Autodesk Inventor part; units mm, degrees
ref_plane "YZ Plane" through (0, 0, 0) normal (1, 0, 0) x (0, 1, 0)
ref_plane "XZ Plane" through (0, 0, 0) normal (0, 1, 0) x (-1, 0, 0)
ref_plane "XY Plane" through (0, 0, 0) normal (0, 0, 1) x (1, 0, 0)
sketch "スケッチ2" plane through (-42.95, -23.5, 0) normal (0, -1, 0) x (1, 0, 0)
  line L0 (0, 0) -> (25.9, 5) construction
  line L1 (0, 5) -> (25.9, 5)
  line L2 (12.95, 5) -> (12.95, 0) construction
  line L3 (0, 0) -> (25.9, 0)
  line L4 (0, 0) -> (0, 5)
  line L5 (0, 2.5) -> (25.9, 2.5) construction
  line L6 (25.9, 0) -> (25.9, 5)
  point P0 (42.95, 0)
  point P1 (2.95, 2.5)
  point P2 (22.95, 2.5)
  dimension "d176" = 20
sketch "スケッチ1" plane through (0, 0, 0) normal (0, 0, 1) x (1, 0, 0)
  line L0 (-72.5, 26.5) -> (-45, 26.5) construction
  line L1 (72.5, 26.5) -> (72.5, 10.5) construction
  line L2 (-72.5, -26.5) -> (-72.5, 10.5)
  line L3 (-72.5, 26.5) -> (72.5, -26.5) construction
  line L4 (72.5, 26.5) -> (-72.5, -26.5) construction
  line L5 (2.5, 26.5) -> (2.5, 10.5)
  line L6 (2.5, 10.5) -> (4.6, 10.5) construction
  line L7 (2.5, 26.5) -> (72.5, 26.5) construction
  line L8 (72.5, 10.5) -> (72.5, -26.5)
  line L9 (70, 10.5) -> (70, -26) construction
  circle A0 centre (67.5, 5.5) radius 1.55
  line L10 (-31.25, 26.5) -> (-31.25, 31.5)
  line L11 (-31.25, 31.5) -> (-11.25, 31.5)
  line L12 (-11.25, 31.5) -> (-11.25, 26.5)
  line L13 (-31.25, 26.5) -> (-11.25, 26.5) construction
  line L14 (-11.25, 26.5) -> (-9.15, 26.5) construction
  arc A1 (-33.35, 26.5) -> (-31.25, 26.5) centre (-32.3, 26.5) ccw
  arc A2 (-11.25, 26.5) -> (-9.15, 26.5) centre (-10.2, 26.5) ccw
  line L15 (-33.35, 26.5) -> (-31.25, 26.5) construction
  line L16 (-9.15, 26.5) -> (2.5, 26.5)
  line L17 (-45.05, -23.5) -> (-42.95, -23.5) construction
  arc A3 (-42.95, -23.5) -> (-45.05, -23.5) centre (-44, -23.5) ccw
  arc A4 (-14.95, -23.5) -> (-17.05, -23.5) centre (-16, -23.5) ccw
  line L18 (-42.95, -23.5) -> (-17.05, -23.5)
  line L19 (-17.05, -23.5) -> (-14.95, -23.5) construction
  line L20 (15, -23.5) -> (45, -23.5) construction
  line L21 (45, -23.5) -> (45, -25) construction
  line L22 (45, -25) -> (15, -25) construction
  line L23 (15, -25) -> (15, -23.5) construction
  line L24 (15, -23.5) -> (45, -25) construction
  line L25 (45, -23.5) -> (15, -25) construction
  line L26 (14.95, -23.45) -> (45.05, -23.45)
  line L27 (45.05, -23.45) -> (45.05, -25.05) construction
  line L28 (45.05, -25.05) -> (14.95, -25.05)
  line L29 (14.95, -25.05) -> (14.95, -23.45) construction
  line L30 (14.95, -23.45) -> (45.05, -25.05) construction
  line L31 (45.05, -23.45) -> (14.95, -25.05) construction
  line L32 (-45, -23.5) -> (-45, -26.5) construction
  line L33 (-15, -23.5) -> (-15, -26.5) construction
  line L34 (72.5, -8) -> (-72.5, -8) construction
  line L35 (70, -0.5) -> (67.5, -0.5) construction
  line L36 (67.5, -0.5) -> (67.5, -15.5) construction
  line L37 (67.5, -15.5) -> (70, -15.5) construction
  line L38 (70, -15.5) -> (70, -0.5) construction
  line L39 (70, -0.5) -> (67.5, -15.5) construction
  line L40 (67.5, -0.5) -> (70, -15.5) construction
  line L41 (67.45, -0.45) -> (70.05, -0.45)
  line L42 (70.05, -0.45) -> (70.05, -2.55) construction
  line L43 (70.05, -15.55) -> (67.45, -15.55)
  line L44 (67.45, -15.55) -> (67.45, -13.45) construction
  line L45 (67.45, -0.45) -> (70.05, -15.55) construction
  line L46 (70.05, -0.45) -> (67.45, -15.55) construction
  arc A5 (67.45, -0.45) -> (67.45, -2.55) centre (67.45, -1.5) ccw
  arc A6 (70.05, -2.55) -> (70.05, -0.45) centre (70.05, -1.5) ccw
  arc A7 (67.45, -13.45) -> (67.45, -15.55) centre (67.45, -14.5) ccw
  arc A8 (70.05, -15.55) -> (70.05, -13.45) centre (70.05, -14.5) ccw
  line L47 (67.45, -2.55) -> (67.45, -0.45) construction
  line L48 (67.45, -13.45) -> (67.45, -2.55)
  line L49 (70.05, -13.45) -> (70.05, -15.55) construction
  line L50 (70.05, -2.55) -> (70.05, -13.45)
  arc A9 (14.95, -23.45) -> (14.95, -25.05) centre (14.95, -24.25) ccw
  arc A10 (45.05, -25.05) -> (45.05, -23.45) centre (45.05, -24.25) ccw
  circle A11 centre (67.5, -21.5) radius 1.55
  line L51 (-72.5, -26.5) -> (-62.5, -26.5) construction
  line L52 (-15, -26.5) -> (72.5, -26.5)
  line L53 (-45, -26.5) -> (-15, -26.5) construction
  line L54 (-70, 26) -> (-70, -26.5) construction
  line L55 (-65, 26.5) -> (-65, -26.5) construction
  arc A12 (2.5, 10.5) -> (4.6, 10.5) centre (3.55, 10.5) ccw
  line L56 (4.6, 10.5) -> (72.5, 10.5)
  circle A13 centre (67.5, 5.5) radius 3
  circle A14 centre (67.5, -21.5) radius 3
  line L57 (2.5, 5.5) -> (2.5, -18.5)
  line L58 (2.5, -18.5) -> (51.8308, -18.5)
  line L59 (51.8308, -18.5) -> (6.5905, 5.5)
  line L60 (17.2597, 5.5) -> (62.5, 5.5)
  line L61 (62.5, 5.5) -> (62.5, -18.5)
  line L62 (62.5, -18.5) -> (17.2597, 5.5)
  line L63 (-62.5, -18.5) -> (-6.9355, -18.5)
  line L64 (-6.9355, -18.5) -> (-42.1079, 5.5)
  line L65 (-2.5, 21.5) -> (-2.5, -15.4734)
  line L66 (-2.5, -15.4734) -> (-40, 10.1148)
  line L67 (2.5, 10.5) -> (2.5, -26.5) construction
  line L68 (6.5905, 5.5) -> (2.5, 5.5)
  line L69 (2.5, 10.5) -> (72.2455, -26.5) construction
  circle A15 centre (-67.5, -29) radius 1.25
  circle A16 centre (-67.5, -29) radius 3
  circle A17 centre (-67.5, -2) radius 1.5
  circle A18 centre (-67.5, 3) radius 1.5
  circle A19 centre (-67.5, 8) radius 1.5
  line L70 (-67.5, 26.5) -> (-67.5, -26.5) construction
  line L71 (-45.05, -23.5) -> (-45.05, -26.5)
  line L72 (-14.95, -23.5) -> (-14.95, -26.5)
  line L73 (-45, 26.5) -> (-45, 21.5)
  line L74 (-45, 10.5) -> (-72.5, 10.5)
  line L75 (-62.5, 5.5) -> (-42.1079, 5.5)
  line L76 (-40, 21.5) -> (-40, 10.1148)
  line L77 (-72.5, -26.5) -> (-72.5, -34)
  line L78 (-72.5, -34) -> (-62.5, -34)
  line L79 (-62.5, -26.5) -> (-62.5, -34)
  line L80 (-62.5, -26.5) -> (-45, -26.5)
  line L81 (-45, 26.5) -> (-33.35, 26.5)
  line L82 (-45, 21.5) -> (-45, 10.5)
  line L83 (-62.5, 5.5) -> (-62.5, -18.5)
  line L84 (-2.5, -18.5) -> (-45, 10.5) construction
  line L85 (-45.05, 21.5) -> (-45, 21.5)
  line L86 (-40, 21.5) -> (-2.5, 21.5)
  line L87 (-72.5, 10.5) -> (-72.5, 26.5) construction
  point P0 (0, 0)
  point P1 (30, -24.25)
  point P2 (68.75, -8)
  point P3 (-60, 14.6054)
  point P4 (-46.25, 11.0112)
  point P5 (-54.1904, 10.5)
  point P6 (-45.5266, 10.5)
  dimension "d0" = 145
  dimension "d1" = 53
  dimension "d2" = 75
  dimension "d3" = 16
  dimension "d4" = 2.5
  dimension "d5" = 3.1
  dimension "d6" = 2.5
  dimension "d7" = 5
  dimension "d12" = 20
  dimension "d14" = 5
  dimension "d15" = 1.05
  dimension "d16" = 1.05
  dimension "d17" = 70
  dimension "d55" = 1.05
  dimension "d56" = 1.05
  dimension "d74" = 37
  dimension "d107" = 30
  dimension "d108" = 1.5
  dimension "d109" = 0.05
  dimension "d110" = 0.05
  dimension "d116" = 30
  dimension "d124" = 15
  dimension "d125" = 0.05
  dimension "d126" = 0.05
  dimension "d127" = 1.05
  dimension "d128" = 1.05
  dimension "d129" = 1.05
  dimension "d130" = 1.05
  dimension "d132" = 30
  dimension "d134" = 3
  dimension "d135" = 2.5
  dimension "d146" = 5
  dimension "d147" = 20
  dimension "d152" = 1.05
  dimension "d169" = 6
  dimension "d186" = 5
  dimension "d187" = 5
  dimension "d190" = 8
  dimension "d192" = 5
  dimension "d193" = 5
  dimension "d196" = 2.5
  dimension "d200" = 2.5
  dimension "d201" = 6
  dimension "d205" = 2.5
  dimension "d206" = 3
  dimension "d207" = 3
  dimension "d208" = 3
  dimension "d209" = 2.5
  dimension "d211" = 5
  dimension "d212" = 5
  dimension "d213" = 0.05
  dimension "d214" = 0.05
  dimension "d215" = 2.5
  dimension "d216" = 5
  dimension "d217" = 2.5
  dimension "d220" = 18.5
  dimension "d222" = 16
  dimension "d225" = 13.75
  dimension "d226" = 27.5
  dimension "d227" = 5
  dimension "d228" = 5
  dimension "d233" = 7.5
  dimension "d234" = 2.5
  dimension "d235" = 2.5
extrude "押し出し1" add sketch "スケッチ1" along normal blind 5 contours L2 L74 L82 L73 L81 A1 L10 L11 L12 A2 L16 L5 A12 L56 L8 L52 L72 A4 L18 A3 L71 L80 L79 L78 L77
extrude "押し出し2" add sketch "スケッチ1" along normal blind 2 contours A13 | A14 | A16
hole "穴1" at (-40, -23.5, 2.5) at (-20, -23.5, 2.5) direction (0, 1, 0) diameter 2.459 depth 5
chamfer "面取り1" distance 2.5 angle 45 5 edges at (72.5, -26.5, 2.5) (72.5, 10.5, 2.5) (-72.5, -34, 2.5) (-72.5, 10.5, 2.5) (-62.5, -34, 2.5)
fillet "フィレット2" radius 1 11 edges at (-6.9355, -18.5, 2.5) (-2.5, -15.4734, 2.5) (2.5, -18.5, 2.5) (2.5, 5.5, 2.5) (6.5905, 5.5, 2.5) (17.2597, 5.5, 2.5) (62.5, 5.5, 2.5) (62.5, -18.5, 2.5) (51.8308, -18.5, 2.5) (-45, 10.5, 2.5) (-62.5, -26.5, 2.5)
extrude "押し出し4" add sketch "スケッチ1" along normal blind 0.5 contours L68 L59 L58 L57 | L60 L61 L62 | L83 L75 L64 L63 | L65 L66 L76 L86
sketch "スケッチ9" plane through (-45, 26.5, 0) normal (0, 1, 0) x (1, 0, 0)
  line L0 (33.75, 0) -> (33.75, -5)
  line L1 (13.75, 0) -> (13.75, -5)
  line L2 (33.75, 0) -> (13.75, 0)
  line L3 (47.5, 0) -> (35.85, 0)
  point P0 (45, 0)
  point P1 (8.75, -2.5)
  point P2 (38.75, -2.5)
  dimension "d237" = 20
  dimension "d238" = 30
  dimension "d239" = 5
  dimension "d240" = 2.5
  dimension "d241" = 2.5
hole "穴6" at (-36.25, 26.5, 2.5) at (-6.25, 26.5, 2.5) direction (0, -1, 0) diameter 2.459 depth 5
equation "\"d16\" = d15"
equation "\"d55\" = d54"
equation "\"d56\" = d55"
equation "\"d53\" = d15"
equation "\"d54\" = d53"
properties part number "Cockpit_battery_side_frame" material "アセタール樹脂、黒"
Check sheet for the modelled part. Datum: model origin and axes. Units: mm. A direction names the side the tool comes from. Coordinates: 2 decimals unless noted, no trailing zeros. Write each loop counter-clockwise with the first axis right and the second up, starting at its lowest first coordinate (ties: lowest second). Pieces come first, ordered by that corner, then holes.
Item 1: Cross-section at C-C on x = -25.5. Record the boundary of the cut face in (y, z), then the cut area to 3 significant figures.
Numbers:
outline: (-23.5, 0) - (31.5, 0) - (31.5, 5) - (21.5, 5) - (21.5, 0.5) - (0.22, 0.5) - (0.22, 5) - (-5.83, 5) - (-5.83, 0.5) - (-18.5, 0.5) - (-18.5, 5) - (-23.5, 5) - close
area: 122 mm2
Item 2: Access from +Z, -Z, +X, -X, +Y, -Y to the whole of each face (thin tool, end or side, straight path). Record for faces 4 (the face through (-45, 19, 2)), 5 (the face through (-17, 8, 0.5)), 6 (the face through (-45.05, -25, 2)).
Numbers:
face 4: +Z, -Z, -X, +Y
face 5: +Z
face 6: +Z, -Z, -Y
Item 3: Cross-section at A-A on x = 29. Record the boundary of the cut face in (y, z).
Numbers:
outline: (-26.5, 0) - (-25.05, 0) - (-25.05, 5) - (-26.5, 5) - close; (-23.45, 0) - (10.5, 0) - (10.5, 5) - (5.5, 5) - (5.5, 0.5) - (-0.73, 0.5) - (-0.73, 5) - (-6.39, 5) - (-6.39, 0.5) - (-18.5, 0.5) - (-18.5, 5) - (-23.45, 5) - close
Item 4: Depth check by flat-ended pin: pin 1 Ø2 at (x, z) = (15, 3.5) entering from +Y; pin 2 Ø10 at (x, y) = (-23.5, 12) entering from +Z; pin 3 Ø3 at (x, z) = (-40, 2.5) entering from -Y. Enter the tip coordinate at first touch or a pass-through.
Numbers:
pin 1: stops at y = 10.5
pin 2: stops at z = 0.5
pin 3: stops at y = -23.5
Item 5: Scan lines: probe 1 along Y at (x, z) = (16, 4.15); probe 2 along Y at (x, z) = (3.5, 1.15); probe 3 along X at (y, z) = (24.25, 2.5). Record each from-to range of solid material in increasing order.
Numbers:
probe 1: y = -26.5 to -25.05, -23.45 to -18.5, 0.51 to 10.5
probe 2: y = -26.5 to -18.5, 5.5 to 9.45
probe 3: x = -45 to -37.48, -35.02 to -7.48, -5.02 to 2.5
Item 6: Cross-section at B-B on y = 20. Record the boundary of the cut face in (x, z).
Numbers:
outline: (-45, 0) - (2.5, 0) - (2.5, 5) - (-2.5, 5) - (-2.5, 0.5) - (-40, 0.5) - (-40, 5) - (-45, 5) - close
Item 7: Mould release check, pull along Y, two halves, no side actions. Record for faces 1 (the face through (-2.5, 4, 3)), 2 (the face through (-72.5, -12, 2)), 3 (the face through (-58, 10.5, 2)): released by +Y, released by -Y, zero draft, split by the parting line, or undercut.
Numbers:
face 1: undercut
face 2: zero draft
face 3: released by +Y
